```python
from build123d import *

# Parameters (mm, degrees)
F0_R     = 25.0538592269
F0_R_2   = 22.1151021615
F1_DEPTH = 30.48
F0_R_3   = 19.05
F2_DEPTH = 20.32
F0_R_4   = 14.2519488642
F3_DEPTH = 15.24
F0_R_5   = 9.329458502
F4_DEPTH = 10.16
F0_R_6   = 4.9036289707
F5_DEPTH = 5.08
F0_R_7   = 2.6620736833
F6_DEPTH = 3.81
F7_DEPTH = 15.24


# Not quite as in the source:
# - a fillet or chamfer that OpenCascade refuses, or shapes differently, is made with other operations: its cross-section is extruded or revolved along the edge and cut away or added


with BuildPart() as f1:
    # F0 (on Front) → F1 (new body)
    with BuildSketch(Plane.XZ):
        Circle(F0_R)
        Circle(F0_R_2, mode=Mode.SUBTRACT)
    extrude(amount=F1_DEPTH)

    # F0 (on Front) → F2 (join)
    with BuildSketch(Plane.XZ):
        Circle(F0_R_2)
        Circle(F0_R_3, mode=Mode.SUBTRACT)
    extrude(amount=F2_DEPTH)

    # F0 (on Front) → F3 (join)
    with BuildSketch(Plane.XZ):
        Circle(F0_R_3)
        Circle(F0_R_4, mode=Mode.SUBTRACT)
    extrude(amount=F3_DEPTH)

    # F0 (on Front) → F4 (join)
    with BuildSketch(Plane.XZ):
        Circle(F0_R_4)
        Circle(F0_R_5, mode=Mode.SUBTRACT)
    extrude(amount=F4_DEPTH)

    # F0 (on Front) → F5 (join)
    with BuildSketch(Plane.XZ):
        Circle(F0_R_5)
        Circle(F0_R_6, mode=Mode.SUBTRACT)
    extrude(amount=F5_DEPTH)

    # F0 (on Front) → F6 (join)
    with BuildSketch(Plane.XZ):
        Circle(F0_R_6)
        Circle(F0_R_7, mode=Mode.SUBTRACT)
    extrude(amount=F6_DEPTH)

    # F0 (on Front) → F7 (join)
    with BuildSketch(Plane.XZ):
        Circle(F0_R_6)
        Circle(F0_R_7, mode=Mode.SUBTRACT)
    extrude(amount=-F7_DEPTH)

    # F8: fillet of radius 5.08 on 6 edges, made by hand

    # F8_s1 → F8_t2 (revolve, cut)
    with BuildSketch(Plane.XY):
        with BuildLine():
            ThreePointArc((25.0538592269, -30.48), (22.9123510534, -28.6054356547), (22.1151021615, -25.87332238))
            Line((22.1151021615, -25.87332238), (22.1151021615, -30.48))
            Line((22.1151021615, -30.48), (25.0538592269, -30.48))
        make_face()
    revolve(axis=Axis((0, -30.48, 0), (0, -1, 0)), mode=Mode.SUBTRACT)

    # F8_s3 → F8_t4 (revolve, cut)
    with BuildSketch(Plane.XY):
        with BuildLine():
            ThreePointArc((22.1151021615, -20.32), (19.8848803892, -18.4469021379), (19.05, -15.6566764319))
            Line((19.05, -15.6566764319), (19.05, -20.32))
            Line((19.05, -20.32), (22.1151021615, -20.32))
        make_face()
    revolve(axis=Axis((0, -20.32, 0), (0, -1, 0)), mode=Mode.SUBTRACT)

    # F8_s5 → F8_t6 (revolve, cut)
    with BuildSketch(Plane.XY):
        with BuildLine():
            ThreePointArc((19.05, -15.24), (15.6415084955, -13.6588259054), (14.2519488642, -10.1678303619))
            Line((14.2519488642, -10.1678303619), (14.2519488642, -15.24))
            Line((14.2519488642, -15.24), (19.05, -15.24))
        make_face()
    revolve(axis=Axis((0, -15.24, 0), (0, -1, 0)), mode=Mode.SUBTRACT)

    # F8_s7 → F8_t8 (revolve, cut)
    with BuildSketch(Plane.XY):
        with BuildLine():
            ThreePointArc((14.2519488642, -10.16), (10.7620930857, -8.6184183396), (9.329458502, -5.082442446))
            Line((9.329458502, -5.082442446), (9.329458502, -10.16))
            Line((9.329458502, -10.16), (14.2519488642, -10.16))
        make_face()
    revolve(axis=Axis((0, -10.16, 0), (0, -1, 0)), mode=Mode.SUBTRACT)

    # F8_s9 → F8_t10 (revolve, cut)
    with BuildSketch(Plane.XY):
        with BuildLine():
            ThreePointArc((4.9036289707, -3.81), (6.4676819116, -4.7519048812), (8.2637331358, -5.08))
            Line((8.2637331358, -5.08), (4.9036289707, -5.08))
            Line((4.9036289707, -5.08), (4.9036289707, -3.81))
        make_face()
    revolve(axis=Axis((0, -5.08, 0), (0, -1, 0)), mode=Mode.SUBTRACT)

    # F8_s11 → F8_t12 (revolve, cut)
    with BuildSketch(Plane.XY):
        with BuildLine():
            ThreePointArc((2.6620736833, 0.4030311669), (3.2573385105, -1.9830850142), (4.9036289707, -3.81))
            Line((4.9036289707, -3.81), (2.6620736833, -3.81))
            Line((2.6620736833, -3.81), (2.6620736833, 0.4030311669))
        make_face()
    revolve(axis=Axis((0, -3.81, 0), (0, -1, 0)), mode=Mode.SUBTRACT)


solid = f1.part
```
Geometry check sheet. Reference: the model listing, model coordinates, mm. A direction names the side the tool comes from. Round coordinates to 2 decimals unless told otherwise and drop trailing zeros. Loops run counter-clockwise (first coordinate to the right, second up) from the corner with the lowest first, then second, coordinate; pieces in that order, holes last. Notation, with made-up numbers: (3.5, 2.5) -> (43.5, 2.5) arc R17 cw to (43.5, 28.5) -> close; hole circle Ø11 at (30.5, 55.25). An arc over 180 degrees is marked (long way). Use a Markdown table: item, result.
(1) Sectioned sample at D-D (y = -11). Enter the section's corners in (x, z), then the cut area to 3 significant figures.
Calculated:
| item | result |
|---|---|
| outline | circle Ø50.11 at (0, 0); hole circle Ø28.64 at (0, 0) |
| area | 1,330 mm² |
(2) Mould release check, pull along Z, two halves, no side actions. Record for faces 3 (the cylindrical face through (4.68, 7.51, 1.47)), 4 (the flat face through (5.2, 0, 0.4)), 5 (the flat face through (-6, -5.08, -6)): released by +Z, released by -Z, zero draft, split by the parting line, or undercut.
Calculated:
| item | result |
|---|---|
| face 3 | split by the parting line |
| face 4 | zero draft |
| face 5 | undercut |
(3) Scan lines: probe 1 along Z at (x, y) = (0, -23); probe 2 along Z at (x, y) = (0, 10); probe 3 along X at (y, z) = (-13, -6). Record each from-to range of solid material in increasing order.
Calculated:
| item | result |
|---|---|
| probe 1 | -25.05 to -22.12, 22.12 to 25.05 |
| probe 2 | -4.9 to -2.66, 2.66 to 4.9 |
| probe 3 | -24.32 to -13.87, 13.87 to 24.32 |
(4) Sectioned sample at C-C (y = -23). Enter the section's corners in (x, z).
Calculated:
| item | result |
|---|---|
| outline | circle Ø50.11 at (0, 0); hole circle Ø44.23 at (0, 0) |
(5) Set-up check for faces 1 (the flat face through (2, 15.24, -2)), 2 (the cylindrical face through (20.43, -23.06, -8.47)): record each of +Z, -Z, +X, -X, +Y, -Y from which the full face is reachable in a straight line by a thin tool's end or side.
Calculated:
| item | result |
|---|---|
| face 1 | +Z, -Z, +X, -X, +Y |
| face 2 | -Y |
(6) Go/stop test with flat-tipped pins: P1, Ø10, axis at y = -22.5, z = 6.5, coming from the +X side; P2, Ø1.5, axis at x = -13, z = -8, coming from the -Y side; P3, Ø6, axis at x = 15, z = -7, coming from the +Y side. Record where each tip stops, or that it passes through.
Calculated:
| item | result |
|---|---|
| P1 | x = 25.01 |
| P2 | y = -14.01 |
| P3 | y = 0 |
